Check sheet for the drawn part. Datum: minimum x, y, z corner. Units: mm. Round coordinates to 2 decimals unless told otherwise and drop trailing zeros. Write each loop counter-clockwise with the first axis right and the second up, starting at its lowest first coordinate (ties: lowest second). Pieces come first, ordered by that corner, then holes. Notation, with made-up numbers: (9, -30) - (36, -30) arc R32 ccw to (36, 8) - close; hole circle Ø9 at (68.25, 40.25). An arc over 180 degrees is marked (long way). Answer as a JSON object with one key per item and string values.
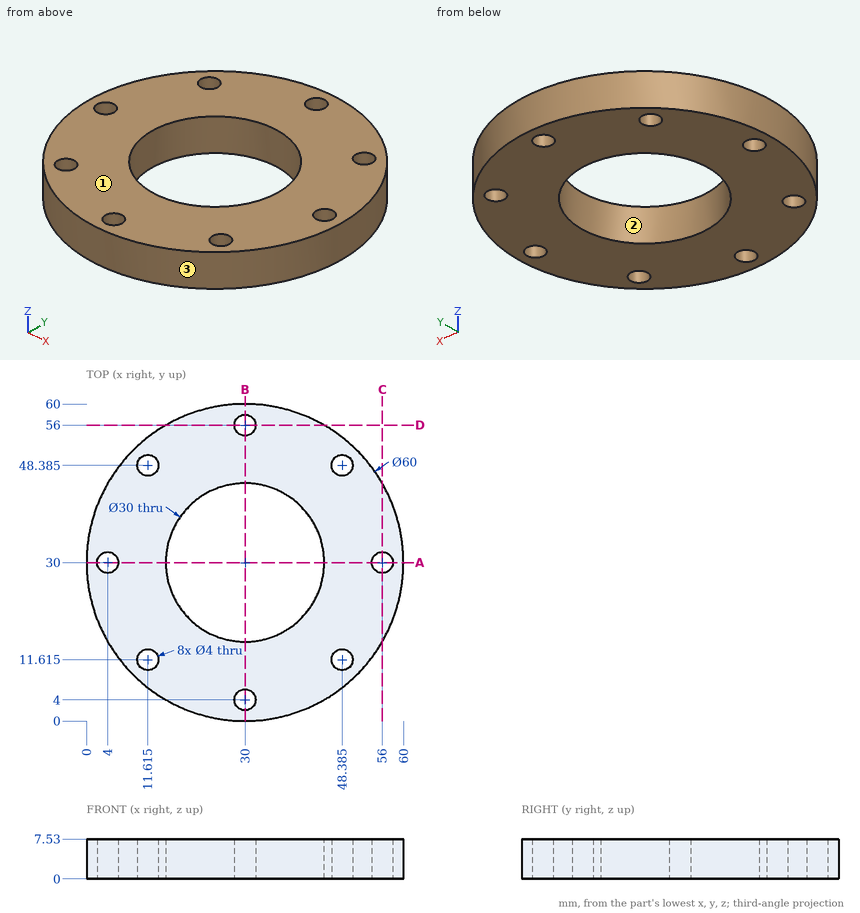
Q1. Gauge pin test, flat ends, axial feed: P1, Ø4, axis at x = 50, z = 1, coming from the -Y side; P2, Ø1, axis at y = 15.5, z = 3.5, coming from the +X side; P3, Ø3, axis at y = 51.5, z = 5.5, coming from the +X side. Record the tip position at first contact, or that the pin passes through.
Geometry check:
{"P1": "stops at y = 6", "P2": "stops at x = 56.53", "P3": "stops at x = 52.36"}
Q2. Section check C-C, the plane x = 56. Record the cut outline in (y, z).
Geometry check:
{"outline": "(15.03, 0) - (28, 0) - (28, 7.53) - (15.03, 7.53) - close; (32, 0) - (44.97, 0) - (44.97, 7.53) - (32, 7.53) - close"}
Q3. Material ranges on line 1 along Y through (x, z) = (30, 4.25); line 2 along Y through (x, z) = (12.5, 2.25); line 3 along Y through (x, z) = (55, 6.5), recorded low to high. Write a range as [from, to].
Geometry check:
{"line 1": "y = [0, 2], [6, 15], [45, 54], [58, 60]", "line 2": "y = [5.63, 9.82], [13.41, 46.59], [50.18, 54.37]", "line 3": "y = [13.42, 28.27], [31.73, 46.58]"}
Q4. Section check A-A, the plane y = 30. Record the cut outline in (x, z), then the cut area to 3 significant figures.
Geometry check:
{"outline": "(0, 0) - (2, 0) - (2, 7.53) - (0, 7.53) - close; (6, 0) - (15, 0) - (15, 7.53) - (6, 7.53) - close; (45, 0) - (54, 0) - (54, 7.53) - (45, 7.53) - close; (58, 0) - (60, 0) - (60, 7.53) - (58, 7.53) - close", "area": "166 mm2"}
Q5. Release check for a two-part mould opening along Y. For the marked faces 1, 2 and 3 record: released by +Y, released by -Y, zero draft, split by the parting line, or undercut.
Geometry check:
{"face 1": "zero draft", "face 2": "undercut", "face 3": "split by the parting line"}
